Verification items for this drawing (mm, ordinates from the low corner). Give positions to 0.01 mm unless a question says otherwise; leave off trailing zeros. Loops run counter-clockwise (first coordinate to the right, second up) from the corner with the lowest first, then second, coordinate; pieces in that order, holes last. Notation, with made-up numbers: M 12,83.5 L 68,83.5 A33 cw 68,115.5 Z; hole C 62.5,52.5 d1. An arc over 180 degrees is marked long. Answer in a Markdown table with one row per item.
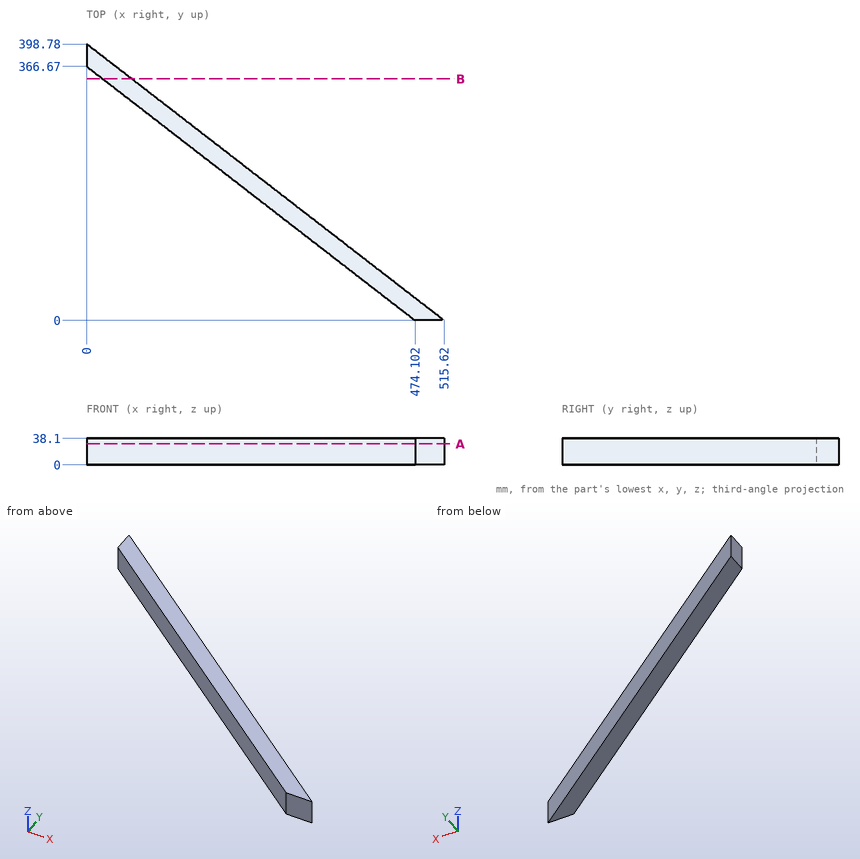
Item 1: Sectioned sample at B-B (y = 348.5). Record the cut outline in (x, z).
Reported:
| item | result |
|---|---|
| outline | M 23.49,0 L 65.01,0 L 65.01,38.1 L 23.49,38.1 Z |
Item 2: Sectioned sample at A-A (z = 30.5). Record the cut outline in (x, y), and give its area (3 significant figures).
Reported:
| item | result |
|---|---|
| outline | M 0,366.67 L 474.1,0 L 515.62,0 L 0,398.78 Z |
| area | 15,900 mm^2 |
Item 3: Go/stop test with flat-tipped pins: pin 1 (6 mm diameter, centred on y = 132.5, z = 23, fed in from +X); pin 2 (2 mm diameter, centred on x = 324, z = 25, fed in from +Y); pin 3 (2 mm diameter, centred on y = 337, z = 15.5, fed in from +X) (1 decimal). Record where each tip stops, or that it passes through.
Reported:
| item | result |
|---|---|
| pin 1 | stops at x = 348.18 |
| pin 2 | stops at y = 148.97 |
| pin 3 | stops at x = 81.2 |
Item 4: Scan lines: L1, parallel to Y at x = 354, z = 32.5; L2, parallel to X at y = 276.5, z = 17.5; L3, parallel to X at y = 320.5, z = 36 (1 decimal). Record each from-to range of solid material in increasing order. Write a range as [from, to].
Reported:
| item | result |
|---|---|
| L1 | y = [92.89, 125] |
| L2 | x = [116.59, 158.11] |
| L3 | x = [59.7, 101.2] |
